Geometry: final body of the model. Coordinates: model frame, mm. A direction names the side the tool comes from. Round coordinates to 2 decimals unless told otherwise and drop trailing zeros. Write each loop counter-clockwise with the first axis right and the second up, starting at its lowest first coordinate (ties: lowest second). Pieces come first, ordered by that corner, then holes. Notation, with made-up numbers: M -28.75,-23.5 L -20.75,-23.5 A32 ccw -20.75,2.5 Z; hole C 58,-21 d9. An arc over 180 degrees is marked long. Use one line per item in the form item = value. Start each with the question number.
Item 1: Pull-direction query (Z, two-part tool) for faces 1 (the cylindrical face through (0.007, -3.728, 2.647)), 2 (the cylindrical face through (0.007, 8.094, -0.322)), 3 (the flat face through (0.01, -6.92, -1.94)), 4 (the flat face through (0.5, -4, 3)); classes: pulls with the +Z half, pulls with the -Z half, needs draft (parallel to the pull), parting line crosses it, or undercut.
Item 2: Pin query (flat end, axial travel): pin 1 Ø1 at (y, z) = (-5.46, 3.15) entering from +X. Return the tip coordinate at first contact, or that it passes through.
Item 3: Reachability of faces 5 (the flat face through (-0.5, -4, 3)), 6 (the flat face through (0.01, -6.94, 1.95)) from +Z, -Z, +X, -X, +Y, -Y: full face, straight path, thin tool, end or side. Return the list, or none.
Item 4: Section query B-B (y = 1). Return loops of the section in (x, z), and give its area (3 significant figures).
Item 5: Section query A-A (z = -5.5). Return loops of the section in (x, y), and give its area (3 significant figures).
Item 6: Section query D-D (x = -0.2). Return loops of the section in (y, z), and give its area (3 significant figures).
Item 7: Section query C-C (z = 3). Return loops of the section in (x, y), and give its area (3 significant figures).
Item 8: Ray query, probe 1 along Y at (x, z) = (-0.1, -3.15); probe 2 along Z at (x, y) = (0.35, -4.5); probe 3 along Y at (x, z) = (0.25, 3.5). Return the intervals inside material, ascending.
from build123d import *

# Parameters (mm, degrees)
SKETCH1_R                = 0.85
BOSS_EXTRUDE1_DEPTH      = 0.5
BOSS_EXTRUDE1_DEPTH_BACK = 0.5


with BuildPart() as part:
    # Sketch1 → Boss-Extrude1 (new body, two sides)
    with BuildSketch(Plane(origin=(0, 0, 0), x_dir=(0, 0, -1), z_dir=(1, 0, 0))) as boss_extrude1_sk:
        with BuildLine():
            Line((-2.40796943, -7.733801344), (-1.478571429, -6.124036784))
            ThreePointArc((-1.478571429, -6.124036784), (-2.688100389, -3.716233413), (-4.932694682, -5.20696271))
            ThreePointArc((-4.932694682, -5.20696271), (0, 6.2), (4.932694682, -5.20696271))
            ThreePointArc((4.932694682, -5.20696271), (2.688100389, -3.716233413), (1.478571429, -6.124036784))
            Line((1.478571429, -6.124036784), (2.40796943, -7.733801344))
            ThreePointArc((2.40796943, -7.733801344), (0, 8.1), (-2.40796943, -7.733801344))
        make_face()
        with Locations((3.15, -5.455960044)):
            Circle(SKETCH1_R, mode=Mode.SUBTRACT)
        with Locations((-3.15, -5.455960044)):
            Circle(SKETCH1_R, mode=Mode.SUBTRACT)
    extrude(amount=BOSS_EXTRUDE1_DEPTH)
    extrude(boss_extrude1_sk.sketch, amount=-BOSS_EXTRUDE1_DEPTH_BACK)


solid = part.part
Working result:
q1.face_1 = undercut
q1.face_2 = parting line crosses it
q1.face_3 = undercut
q1.face_4 = needs draft
q2.pin_1 = through
q3.face_5 = +Z, -Z, -X, +Y, -Y
q3.face_6 = +X, -X, -Y
q4.outline = M -0.5,-8.04 L 0.5,-8.04 L 0.5,-6.59 L -0.5,-6.59 Z; M -0.5,6.59 L 0.5,6.59 L 0.5,8.04 L -0.5,8.04 Z
q4.area = 2.91 mm²
q5.outline = M -0.5,-5.95 L 0.5,-5.95 L 0.5,-4.52 L -0.5,-4.52 Z; M -0.5,3.38 L 0.5,3.38 L 0.5,5.95 L -0.5,5.95 Z
q5.area = 4.00 mm²
q6.outline = M -7.73,-2.41 A8.1 ccw long -7.73,2.41 L -6.12,1.48 A1.8 ccw long -5.21,4.93 A6.77 cw long -5.21,-4.93 A1.8 ccw long -6.12,-1.48 Z; hole C -5.46,-3.15 d1.7; hole C -5.46,3.15 d1.7
q6.area = 70.6 mm²
q7.outline = M -0.5,-7.52 L 0.5,-7.52 L 0.5,-6.29 L -0.5,-6.29 Z; M -0.5,-4.62 L 0.5,-4.62 L 0.5,-3.66 L -0.5,-3.66 Z; M -0.5,5.5 L 0.5,5.5 L 0.5,7.52 L -0.5,7.52 Z
q7.area = 4.21 mm²
q8.probe_1 = -7.46 to -6.31, -4.61 to -3.66, 5.42 to 7.46
q8.probe_2 = -6.73 to -5.51, -4.68 to -1.62, 1.62 to 4.68, 5.51 to 6.73
q8.probe_3 = -7.3 to -6.23, -4.68 to -3.69, 5.23 to 7.3
